from build123d import *

# Parameters (mm, degrees)
F0_W          = 75
F0_H          = 200
F1_DEPTH      = 10
F2_R          = 15
F3_DEPTH      = 219
F3_DEPTH_BACK = 25
F4_R          = 20


# Not quite as in the source:
# - an extrude ends at something that could not be found from the text; its depth is read off the source's solid


with BuildPart() as f1:
    # F0 (on Front) → F1 (new body)
    with BuildSketch(Plane.XZ):
        Rectangle(F0_W, F0_H)
    extrude(amount=F1_DEPTH)

    # F2 (on Front) → F3 (cut, two sides)
    with BuildSketch(Plane.XZ) as f3_sk:
        with Locations((0, 60)):
            Circle(F2_R)
    extrude(amount=-F3_DEPTH, mode=Mode.SUBTRACT)
    extrude(f3_sk.sketch, amount=F3_DEPTH_BACK, mode=Mode.SUBTRACT)

    # F4
    f4_edges = [f1.edges().sort_by_distance(p)[0] for p in [
        (-37.5, -5, 100),
        (37.5, -5, 100),
    ]]
    fillet(f4_edges, radius=F4_R)


solid = f1.part
Can you work these out from the model? Positions are in its coordinate system, mm. Coordinates: 2 decimals unless noted, no trailing zeros. Write each loop counter-clockwise with the first axis right and the second up, starting at its lowest first coordinate (ties: lowest second). Pieces come first, ordered by that corner, then holes. Notation, with made-up numbers: (71.25, -10) -> (128.25, -10) arc R35 cw to (128.25, 29) -> close; hole circle Ø10 at (6, 68.5). An arc over 180 degrees is marked (long way). Write item = value, one per line.
(1) For pin 1 (1.5 mm diameter, centred on x = 4, z = -11.5, fed in from +Y), with a flat end and sliding along its axis, tell me the tip position at first contact or that it passes through.
Verdict:
pin_1 = 0
(2) If I drill on probe 1 along Z at (x, y) = (0, -1.75); probe 2 along X at (y, z) = (-2.25, 60); probe 3 along Z at (x, y) = (5, -4.75), over which ranges is the centre line in solid material (lowest first)?
Verdict:
probe_1 = -100 to 45, 75 to 100
probe_2 = -37.5 to -15, 15 to 37.5
probe_3 = -100 to 45.86, 74.14 to 100
(3) Imagine slicing it at D-D (x = 29). Please give me the cut outline in (y, z).
Verdict:
outline = (-10, -100) -> (0, -100) -> (0, 96.36) -> (-10, 96.36) -> close
(4) Imagine slicing it at A-A (z = 60). Please give me the cut outline in (x, y).
Verdict:
outline = (-37.5, -10) -> (-15, -10) -> (-15, 0) -> (-37.5, 0) -> close; (15, -10) -> (37.5, -10) -> (37.5, 0) -> (15, 0) -> close
(5) Thinking about a two-plate mould opening in Z: for faces 1 (the face through (31.486, -5.07, 94.297)), 2 (the face through (-3.252, -4.93, 45.357)), 3 (the face through (-1, 0, 1)), which applies, +Z half, -Z half, draft (parallel to the pull), parting line (faces both ways), or undercut?
Verdict:
face_1 = +Z half
face_2 = undercut
face_3 = draft
(6) Imagine slicing it at C-C (y = -6.25). Please give me the cut outline in (x, z).
Verdict:
outline = (-37.5, -100) -> (37.5, -100) -> (37.5, 80) arc R20 ccw to (17.5, 100) -> (-17.5, 100) arc R20 ccw to (-37.5, 80) -> close; hole circle Ø30 at (0, 60)
(7) Imagine slicing it at B-B (x = 0). Please give me the cut outline in (y, z).
Verdict:
outline = (-10, -100) -> (0, -100) -> (0, 45) -> (-10, 45) -> close; (-10, 75) -> (0, 75) -> (0, 100) -> (-10, 100) -> close
